```python
from build123d import *

# Parameters (mm, degrees)
F0_W     = 253
F0_H     = 38
F1_DEPTH = 1.2
F0_W_2   = 280
F0_H_2   = 80
F0_W_3   = 268.5
F0_H_3   = 68.5
F2_DEPTH = 24
F4_SIZE  = 0.5


with BuildPart() as f1:
    # F0 (on Top) → F1 (new body)
    with BuildSketch(Plane.XY):
        with Locations((-39.450533092, 8.8307528198)):
            Rectangle(F0_W, F0_H)
    extrude(amount=-F1_DEPTH)


with BuildPart() as f1b:
    # F0 (on Top) → F1, piece 2 (new body)
    with BuildSketch(Plane.XY):
        with Locations((-39.450533092, 1.3307528198)):
            Rectangle(F0_W_2, F0_H_2)
        with Locations((-39.450533092, 1.3307528198)):
            Rectangle(F0_W_3, F0_H_3, mode=Mode.SUBTRACT)
    extrude(amount=-F1_DEPTH)


with BuildPart() as f2:
    # F0 (on Top) → F2 (new body)
    with BuildSketch(Plane.XY):
        with Locations((-39.450533092, 1.3307528198)):
            Rectangle(F0_W_3, F0_H_3)
        Polygon((-165.950533092, -10.1692471802), (-165.950533092, 27.8307528198), (87.049466908, 27.8307528198), (87.049466908, -10.1692471802), (87.049466908, -25.1692471802), (-165.950533092, -25.1692471802), align=None, mode=Mode.SUBTRACT)
    extrude(amount=-F2_DEPTH)

    # F3: union F1, F1b
    add(f1.part)
    add(f1b.part)

    # F4
    f4_edges = [f2.edges().sort_by_distance(p)[0] for p in [
        (-39.450533, -38.669247, 0),
        (-179.450533, 1.330753, 0),
        (-39.450533, 41.330753, 0),
        (100.549467, 1.330753, 0),
        (-39.450533, -10.169247, 0),
        (87.049467, -17.669247, 0),
        (-39.450533, -25.169247, 0),
        (-165.950533, -17.669247, 0),
    ]]
    chamfer(f4_edges, length=F4_SIZE)


solid = f2.part
```
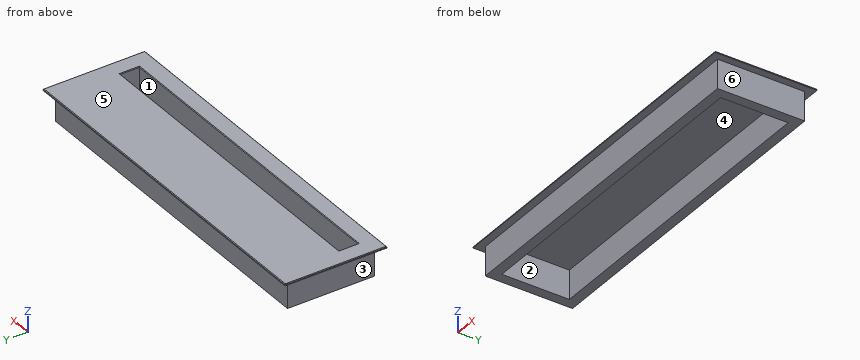
The listing builds one solid part. Answer for the finished solid, in the listing's coordinates (mm). Face numbers are marked on the shaded views. A direction names the side the tool comes from. Coordinates: 2 decimals unless noted, no trailing zeros. Loops run counter-clockwise (first coordinate to the right, second up) from the corner with the lowest first, then second, coordinate; pieces in that order, holes last. Notation, with made-up numbers: (-38.5, 13) -> (-34.5, 13) arc R32 cw to (-34.5, 41) -> close; hole circle Ø9 at (56, 35.5). An arc over 180 degrees is marked (long way). Use one line per item in the form item = value. Start each with the question number.
Item 1: The part is cut by section B-B on x = -127. Determine the outline of the cut face in (y, z), then the cut area to 3 significant figures.
Item 2: The part is cut by section A-A on z = -7.25. Determine the outline of the cut face in (x, y).
Item 3: Flat-ended cylindrical pins translate along their axes: pin 1 Ø12 at (x, y) = (-128.5, 8) entering from -Z; pin 2 Ø4 at (y, z) = (28, -6) entering from -X; pin 3 Ø3 at (y, z) = (-6.5, -11) entering from +X; pin 4 Ø10 at (x, y) = (36.5, -10.5) entering from +Z. Find the tip coordinate at first contact, or state that the pin passes through.
Item 4: The mould has two halves that part along X. Classify the marked faces 4, 5 and 6: released by +X, released by -X, zero draft, split by the parting line, or undercut.
Item 5: Consider L1, parallel to Y at x = -164, z = -11.75; L2, parallel to X at y = 25.5, z = -5.5; L3, parallel to X at y = -26.5, z = -10.25. Determine where each line is inside the solid, lowest interval first. Write a range as [from, to].
Item 6: A tool of negligible diameter and unlimited length cuts with its end or side. For the marked faces 1, 2 and 3, from which of +Z, -Z, +X, -X, +Y, -Y can it reach the whole face along a straight path? Write none if from no direction.
Item 7: The part is cut by section C-C on y = 7.5. Determine the outline of the cut face in (x, z).
Answer key:
q1.outline = (-38.67, -1.2) -> (-32.92, -1.2) -> (-32.92, -24) -> (-25.17, -24) -> (-25.17, -0.5) -> (-25.67, 0) -> (-38.17, 0) -> (-38.67, -0.5) -> close; (-10.17, -1.2) -> (27.83, -1.2) -> (27.83, -24) -> (35.58, -24) -> (35.58, -1.2) -> (41.33, -1.2) -> (41.33, -0.5) -> (40.83, 0) -> (-9.67, 0) -> (-10.17, -0.5) -> close
q1.area = 431 mm2
q2.outline = (-173.7, -32.92) -> (94.8, -32.92) -> (94.8, 35.58) -> (-173.7, 35.58) -> close; hole (-165.95, -25.17) -> (87.05, -25.17) -> (87.05, 27.83) -> (-165.95, 27.83) -> close
q3.pin_1 = -1.2
q3.pin_2 = -173.7
q3.pin_3 = 94.8
q3.pin_4 = 0
q4.face_4 = undercut
q4.face_5 = zero draft
q4.face_6 = released by +X
q5.L1 = [-32.92, -25.17], [27.83, 35.58]
q5.L2 = [-173.7, -165.95], [87.05, 94.8]
q5.L3 = [-173.7, 94.8]
q6.face_1 = +Z, -Z
q6.face_2 = -Z
q6.face_3 = -Z, -X, +Y, -Y
q7.outline = (-179.45, -1.2) -> (-173.7, -1.2) -> (-173.7, -24) -> (-165.95, -24) -> (-165.95, -1.2) -> (87.05, -1.2) -> (87.05, -24) -> (94.8, -24) -> (94.8, -1.2) -> (100.55, -1.2) -> (100.55, -0.5) -> (100.05, 0) -> (-178.95, 0) -> (-179.45, -0.5) -> close
